Could you check a few things on this model? Use its own coordinates, in mm. A direction names the side the tool comes from. Give positions to 0.01 mm unless a question says otherwise; leave off trailing zeros. Loops run counter-clockwise (first coordinate to the right, second up) from the corner with the lowest first, then second, coordinate; pieces in that order, holes last. Notation, with made-up numbers: (83, 60.5) - (117, 60.5) arc R4 cw to (117, 66.5) - close; hole circle Ø4 at (-25, 67.25). An arc over 180 degrees is marked (long way). Use CSV: the item, a comma, the result in double quotes.
from build123d import *

# Parameters (mm, degrees)
F0_W     = 6.3500026588
F0_H     = 558.8
F0_W_2   = 6.35
F0_H_2   = 25.4
F0_W_3   = 6.3499973412
F1_DEPTH = 25.4
F2_W     = 6.35
F2_H     = 6.35
F3_DEPTH = 609.601


with BuildPart() as f1:
    # F0 (on Right) → F1 (new body)
    with BuildSketch(Plane.YZ):
        with Locations((3.1750013294, -279.4)):
            Rectangle(F0_W, F0_H)
        with Locations((9.5250026588, 12.7)):
            Rectangle(F0_W_2, F0_H_2)
        with Locations((9.5250026588, -279.4)):
            Rectangle(F0_W_2, F0_H)
        with Locations((15.8750013294, -279.4)):
            Rectangle(F0_W_3, F0_H)
        with Locations((9.5250026588, -571.5)):
            Rectangle(F0_W_2, F0_H_2)
    extrude(amount=F1_DEPTH)

    # F2 (on face) → F3 (cut, through all)
    with BuildSketch(Plane.XY.offset(25.4)):
        with Locations((22.225, 9.5250026588)):
            Rectangle(F2_W, F2_H)
    extrude(amount=-F3_DEPTH, mode=Mode.SUBTRACT)


solid = f1.part
1) I need wall thicknesses on line 1 along Y through (x, z) = (24, -195); line 2 along Z through (x, y) = (22.25, 3.25); line 3 along X through (y, z) = (11.5, -160). Which ranges of each line are inside material? Lowest first, please.
Answer below:
line 1,"y = 0 to 6.35, 12.7 to 19.05"
line 2,"z = -558.8 to 0"
line 3,"x = 0 to 19.05"
2) Which directions (+Z, -Z, +X, -X, +Y, -Y) give clear straight access to the entire face, cutting with the end or side of a thin tool? Please do faces 1 (the flat face through (9, 12.7, -572)), 2 (the flat face through (9, 6.35, 13)), 3 (the flat face through (9, 6.35, -572)).
Answer below:
face 1,"-Z, +X, -X, +Y"
face 2,"+Z, +X, -X, -Y"
face 3,"-Z, +X, -X, -Y"
3) Suppose I cut it at A-A (z = -240). Please give me the cut outline in (x, y), plus the area to 3 significant figures.
Answer below:
outline,"(0, 0) - (25.4, 0) - (25.4, 6.35) - (19.05, 6.35) - (19.05, 12.7) - (25.4, 12.7) - (25.4, 19.05) - (0, 19.05) - close"
area,"444 mm2"
4) Suppose I cut it at C-C (y = 15.75). Please give me the cut outline in (x, z), plus the area to 3 significant figures.
Answer below:
outline,"(0, -558.8) - (25.4, -558.8) - (25.4, 0) - (0, 0) - close"
area,"14,200 mm2"
5) Suppose I cut it at B-B (x = 10.75). Please give me the cut outline in (y, z).
Answer below:
outline,"(0, -558.8) - (6.35, -558.8) - (6.35, -584.2) - (12.7, -584.2) - (12.7, -558.8) - (19.05, -558.8) - (19.05, 0) - (12.7, 0) - (12.7, 25.4) - (6.35, 25.4) - (6.35, 0) - (0, 0) - close"
6) I'm going to push flat-ended pins straight in: P1, Ø9.5, axis at x = 12, z = 12, coming from the +Y side; P2, Ø3, axis at x = 11, y = 2.5, coming from the -Z side; P3, Ø4, axis at y = 8.5, z = -98, coming from the +X side. Where does each tip first touch, or does it pass through?
Answer below:
P1,"stops at y = 12.7"
P2,"stops at z = -558.8"
P3,"stops at x = 19.05"
